Check sheet for the modelled part. Datum: model origin and axes. Units: mm. A direction names the side the tool comes from. Give positions to 0.01 mm unless a question says otherwise; leave off trailing zeros. Loops run counter-clockwise (first coordinate to the right, second up) from the corner with the lowest first, then second, coordinate; pieces in that order, holes last. Notation, with made-up numbers: M 12.5,61 L 37.5,61 A15 ccw 37.5,82 Z; hole C -23,17 d9. An arc over 180 degrees is marked long. Put each result on its own line as item: value. Start each with the question number.
```python
from build123d import *

# Parameters (mm, degrees)
SKETCH_2_W          = 95
SKETCH_2_H          = 65
EXTRUDE_1_DEPTH     = 30
FILLET_1_R          = 5
SKETCH_3_R          = 1.5
CUT_EXTRUDE_1_DEPTH = 10
SKETCH_4_W          = 44.622650634
SKETCH_4_H          = 17.76241433
CUT_EXTRUDE_2_DEPTH = 3


with BuildPart() as part:
    # 草图2 → 凸台-拉伸1 (new body)
    with BuildSketch(Plane(origin=(0, 0, 0), x_dir=(1, 0, 0), z_dir=(0, 1, 0))):
        Rectangle(SKETCH_2_W, SKETCH_2_H)
    extrude(amount=EXTRUDE_1_DEPTH)

    # 圆角1
    fillet_1_edges = [part.edges().sort_by_distance(p)[0] for p in [
        (47.5, 15, 32.5),
        (-47.5, 15, 32.5),
        (-47.5, 15, -32.5),
        (47.5, 15, -32.5),
    ]]
    fillet(fillet_1_edges, radius=FILLET_1_R)

    # 草图3 → 切除-拉伸1 (cut)
    with BuildSketch(Plane.XZ):
        with Locations(Location((-40.661720084, 23, 0), (0, 0, 270))):
            Circle(SKETCH_3_R)
        with Locations(Location((-40.661720084, -23, 0), (0, 0, 270))):
            Circle(SKETCH_3_R)
        with Locations(Location((14.338279916, 23, 0), (0, 0, 270))):
            Circle(SKETCH_3_R)
        with Locations(Location((14.338279916, -23, 0), (0, 0, 270))):
            Circle(SKETCH_3_R)
    extrude(amount=-CUT_EXTRUDE_1_DEPTH, mode=Mode.SUBTRACT)

    # 草图4 → 切除-拉伸2 (cut)
    with BuildSketch(Plane(origin=(47.5, 0, 0), x_dir=(0, 0, -1), z_dir=(1, 0, 0))):
        with Locations((-0.211139555, 14.091574869)):
            Rectangle(SKETCH_4_W, SKETCH_4_H)
    extrude(amount=-CUT_EXTRUDE_2_DEPTH, mode=Mode.SUBTRACT)


solid = part.part
```
Q1. Thickness scan on line 1 along X through (y, z) = (4.5, -23); line 2 along X through (y, z) = (15.5, -3.5); line 3 along X through (y, z) = (24.75, -29). Record the ranges inside material, lowest first. Write a range as [from, to].
Q2. Depth check by flat-ended pin: P1, Ø1.8, axis at x = -40.66, z = 23, coming from the -Y side; P2, Ø5.5, axis at y = 14.5, z = -6, coming from the +X side; P3, Ø2.5, axis at x = 45.5, y = 17.5, coming from the +Z side. Enter the tip coordinate at first touch or a pass-through.
Q3. Section check C-C, the plane y = 8.25. Record the cut outline in (x, z).
Q4. Section check B-B, the plane z = 12. Record the cut outline in (x, y), then the cut area to 3 significant figures.
Q5. Access from +Z, -Z, +X, -X, +Y, -Y to the whole of each face (thin tool, end or side, straight path). Record for faces 5 (the face through (-47.5, 15, 0)), 6 (the face through (15.826, 4.93, -22.805)), 7 (the face through (46, 14, 22.522)).
Q6. Mould release check, pull along X, two halves, no side actions. Record for faces 1 (the face through (-41, 10, 23)), 2 (the face through (-41, 10, -23)), 3 (the face through (-1, 0, 0)), 4 (the face through (46, 15.21, 31.07)): pulls with the +X half, pulls with the -X half, needs draft (parallel to the pull), parting line crosses it, or undercut.
Q7. Section check A-A, the plane y = 21. Record the cut outline in (x, z).
Found:
1. line 1: x = [-47.5, -42.16], [-39.16, 12.84], [15.84, 47.5]
1. line 2: x = [-47.5, 44.5]
1. line 3: x = [-47.27, 47.27]
2. P1: stops at y = 10
2. P2: stops at x = 44.5
2. P3: stops at z = 32.18
3. outline: M -47.5,-27.5 A5 ccw -42.5,-32.5 L 42.5,-32.5 A5 ccw 47.5,-27.5 L 47.5,-22.1 L 44.5,-22.1 L 44.5,22.52 L 47.5,22.52 L 47.5,27.5 A5 ccw 42.5,32.5 L -42.5,32.5 A5 ccw -47.5,27.5 Z; hole C -40.66,-23 d3; hole C -40.66,23 d3; hole C 14.34,-23 d3; hole C 14.34,23 d3
4. outline: M -47.5,0 L 47.5,0 L 47.5,5.21 L 44.5,5.21 L 44.5,22.97 L 47.5,22.97 L 47.5,30 L -47.5,30 Z
4. area: 2,800 mm^2
5. face 5: +Z, -Z, -X, +Y, -Y
5. face 6: -Y
5. face 7: +X
6. face 1: undercut
6. face 2: undercut
6. face 3: needs draft
6. face 4: pulls with the +X half
7. outline: M -47.5,-27.5 A5 ccw -42.5,-32.5 L 42.5,-32.5 A5 ccw 47.5,-27.5 L 47.5,-22.1 L 44.5,-22.1 L 44.5,22.52 L 47.5,22.52 L 47.5,27.5 A5 ccw 42.5,32.5 L -42.5,32.5 A5 ccw -47.5,27.5 Z
